```python
from build123d import *

# Parameters (mm, degrees)
SKETCH2_W               = 50
SKETCH2_H               = 20
BOSS_EXTRUDE1_DEPTH     = 684.5
CUT_EXTRUDE1_DEPTH      = 690.708998128
CUT_EXTRUDE1_DEPTH_BACK = 690.708998128
SKETCH3_R               = 7
SKETCH4_R               = 7
CUT_EXTRUDE2_DEPTH      = 14


with BuildPart() as part:
    # Sketch2 → Boss-Extrude1 (new body)
    with BuildSketch(Plane.XY):
        with Locations((-57.208588957, 18.374233129)):
            Rectangle(SKETCH2_W, SKETCH2_H)
    extrude(amount=BOSS_EXTRUDE1_DEPTH)

    # Sketch3 → Cut-Extrude1 (cut, two sides: drawn at the far end of the back side and taken through both)
    with BuildSketch(Plane(origin=(0, 28.374233129, 0), x_dir=(1, 0, 0), z_dir=(0, 1, 0)).offset(-CUT_EXTRUDE1_DEPTH_BACK)):
        with Locations(Location((-57.208588957, -673.5, 0), (0, 0, 270))):
            Circle(SKETCH3_R)
        with Locations(Location((-57.208588957, -655.1, 0), (0, 0, 270))):
            Circle(SKETCH3_R)
    extrude(amount=CUT_EXTRUDE1_DEPTH + CUT_EXTRUDE1_DEPTH_BACK, mode=Mode.SUBTRACT)

    # Sketch4 → Cut-Extrude2 (cut)
    with BuildSketch(Plane(origin=(0, 0, 0), x_dir=(-1, 0, 0), z_dir=(0, 0, -1))):
        with Locations((57.208588957, 18.374233129)):
            Circle(SKETCH4_R)
    extrude(amount=-CUT_EXTRUDE2_DEPTH, mode=Mode.SUBTRACT)


solid = part.part
```
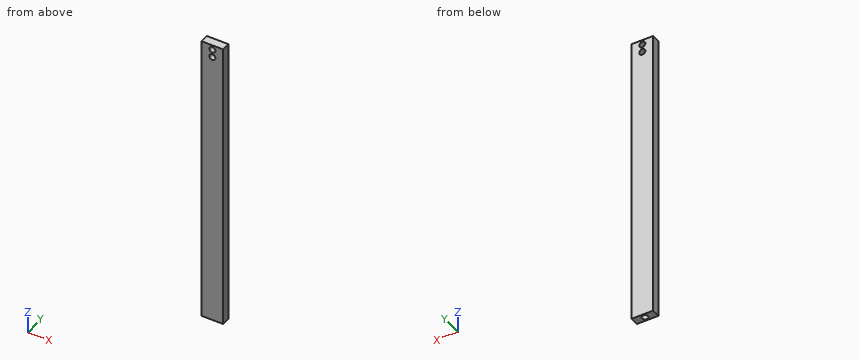
Can you work these out from the model? Positions are in its coordinate system, mm. Give positions to 0.01 mm unless a question says otherwise; leave off trailing zeros. Loops run counter-clockwise (first coordinate to the right, second up) from the corner with the lowest first, then second, coordinate; pieces in that order, holes last. Notation, with made-up numbers: M 7,-6 L 54,-6 A22 ccw 54,30 Z; hole C 41,-37.75 d10. An arc over 180 degrees is marked long. Use one line per item in the form item = value. Start each with the question number.
(1) I want a section at A-A, the plane z = 655.1. Write out the boundary of the cut face in (x, y), and give its area (3 significant figures).
(2) Please list where these lines run through material, in increasing order: line 1 (X direction, y = 23, z = 655.1); line 2 (Z direction, x = -63.5, y = 19.75); line 3 (Z direction, x = -62, y = 27.5).
(3) I'm going to push a flat-ended pin straight in: P1, Ø8.5, axis at x = -57.21, y = 18.37, coming from the -Z side. Where does the tip first touch, or does it pass through?
Worked out:
q1.outline = M -82.21,8.37 L -64.21,8.37 L -64.21,28.37 L -82.21,28.37 Z; M -50.21,8.37 L -32.21,8.37 L -32.21,28.37 L -50.21,28.37 Z
q1.area = 720 mm²
q2.line_1 = -82.21 to -64.21, -50.21 to -32.21
q2.line_2 = 14 to 652.03, 658.17 to 670.43, 676.57 to 684.5
q2.line_3 = 0 to 650, 660.2 to 668.4, 678.6 to 684.5
q3.P1 = 14
